The listing builds one solid part. Answer for the finished solid, in the listing's coordinates (mm). A direction names the side the tool comes from. Coordinates: 2 decimals unless noted, no trailing zeros. Loops run counter-clockwise (first coordinate to the right, second up) from the corner with the lowest first, then second, coordinate; pieces in that order, holes last. Notation, with made-up numbers: (70.5, -38.75) - (79.5, -38.75) arc R24 cw to (79.5, -7.75) - close; hole circle Ø2 at (67, -16.5). An arc over 180 degrees is marked (long way). Write each question's results on one line, items separated by ' | '. Start each with the question number.
(1) Consider line 1 (X direction, y = -3.5, z = -0.05); line 2 (X direction, y = 4.5, z = -0.5). Determine where each line is inside the solid, lowest interval first. Write a range as from..to.
(2) For faces 1 (the flat face through (0, -21.9, 0)), 2 (the cylindrical face through (-0.27, -10.8, 1.22)), 3 (the cylindrical face through (-0.27, 7.06, -1.22)), determine the directions among +Z, -Z, +X, -X, +Y, -Y from which every point of the face is accessible in a straight line to the end or side of a thin tool.
(3) Find section A-A on y = -10. Determine the outline of the cut face in (x, z).
Autodesk Inventor part; units mm, degrees
ref_plane "YZ Plane" through (0, 0, 0) normal (1, 0, 0) x (0, 1, 0)
ref_plane "XZ Plane" through (0, 0, 0) normal (0, 1, 0) x (-1, 0, 0)
ref_plane "XY Plane" through (0, 0, 0) normal (0, 0, 1) x (1, 0, 0)
sketch "Sketch1" plane through (0, 0, 0) normal (0, 1, 0) x (-1, 0, 0)
  line L0 (-1.5, 1.5) -> (1.5, 1.5)
  line L1 (1.5, 1.5) -> (1.5, -1.5)
  line L2 (1.5, -1.5) -> (-1.5, -1.5)
  line L3 (-1.5, -1.5) -> (-1.5, 1.5)
  line L4 (-1.5, 1.5) -> (1.5, -1.5) construction
  line L5 (1.5, 1.5) -> (-1.5, -1.5) construction
  point P0 (0, 0)
  dimension "d0" = 3
  dimension "d1" = 3
extrude "Extrusion1" add sketch "Sketch1" along normal blind 4.1
sketch "Sketch2" plane through (0, 4.1, 0) normal (0, 1, 0) x (1, 0, 0)
  circle A0 centre (0, 0) radius 1.25
  dimension "d4" = 2.5
extrude "Extrusion2" add sketch "Sketch2" along normal blind 6
sketch "Sketch3" plane through (0, 0, 0) normal (0, -1, 0) x (1, 0, 0)
  circle A0 centre (0, 0) radius 1.25
  dimension "d7" = 2.5
extrude "Extrusion3" add sketch "Sketch3" along normal blind 21.9
thread "Thread1"
thread "Thread2"
sketch "Sketch4" plane through (0, 0, 0) normal (1, 0, 0) x (0, 1, 0)
  line L0 (0, 1.5) -> (4.1, 1.5) construction
  line L1 (4.1, 1.5) -> (4.1, 1.25) construction
  line L2 (4.1, 1.25) -> (10.1, 1.25) construction
  line L3 (10.1, 1.25) -> (10.1, -1.25) construction
  line L4 (10.1, -1.25) -> (4.1, -1.25) construction
  line L5 (4.1, -1.25) -> (4.1, -1.5) construction
  line L6 (4.1, -1.5) -> (0, -1.5) construction
  line L7 (0, -1.5) -> (0, -1.25) construction
  line L8 (0, -1.25) -> (-21.9, -1.25) construction
  line L9 (-21.9, -1.25) -> (-21.9, 1.25) construction
  line L10 (-21.9, 1.25) -> (0, 1.25) construction
  line L11 (0, 1.25) -> (0, 1.5) construction
  line L12 (0, -1.25) -> (0.25, -1.5)
  line L13 (0, -1.25) -> (0.3536, -1.25) construction
  line L14 (0, -1.25) -> (0, -1.5)
  line L15 (0, -1.5) -> (4.1, -1.5)
  line L16 (-28.3, 0) -> (16.5, 0)
  line L17 (0, -1.5) -> (0, -2.5685)
  line L18 (0, -2.5685) -> (0.9588, -2.2088)
  line L19 (0.9588, -2.2088) -> (0.25, -1.5)
  point P0 (0, 0)
  dimension "d15" = 45
revolve "Revolution1" cut sketch "Sketch4" angle 360 about axis through (0, -10, 0) along (0, 1, 0)
properties part number "500-001" material "Steel"
Values:
1) line 1: x = -1.25..1.25 | line 2: x = -1.15..1.15
2) face 1: +Z, -Z, +X, -X, -Y | face 2: -Y | face 3: +Y
3) outline: circle Ø2.5 at (0, 0)
